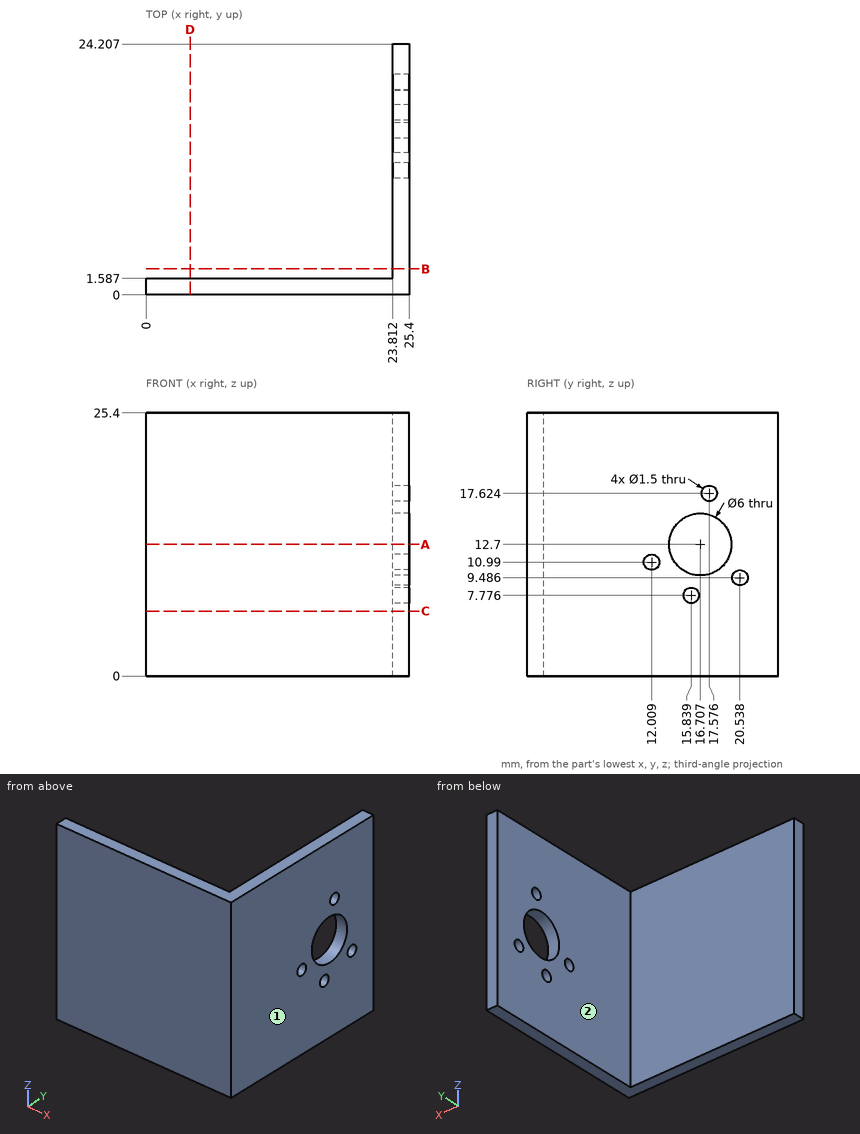
For this review, use the dimensioned drawing (mm, ordinates from the lowest corner) and the shaded views. A direction names the side the tool comes from. Coordinates: 2 decimals unless noted, no trailing zeros. Loops run counter-clockwise (first coordinate to the right, second up) from the corner with the lowest first, then second, coordinate; pieces in that order, holes last.
1. Add section A-A, the plane z = 12.7. Give the boundary of the cut face in (x, y).
2. Add section B-B, the plane y = 2.5. Give the boundary of the cut face in (x, z).
3. Add section D-D, the plane x = 4.25. Give the boundary of the cut face in (y, z).
4. Insertion check: P1, Ø11.5, axis at y = 18, z = 17, coming from the -X side; P2, Ø12, axis at x = 2.5, z = 21.5, coming from the +Y side. Each pin has a flat end and moves straight along its axis. Give the tip position at first contact, or say it passes through.
5. Add section C-C, the plane z = 6.25. Give the boundary of the cut face in (x, y).
6. For line 1 (Y direction, x = 24.6, z = 12.7); line 2 (Y direction, x = 15.5, z = 15); line 3 (X direction, y = 6.5, z = 12.75), list the stretches that pass through material, from the lowest coordinate up.
7. For the marked faces 1 and 2, list the 3-axis set-ups (+Z, -Z, +X, -X, +Y, -Y) from which the entire face can be reached by the end or side of a thin tool; tool diameter is ignored.
Result:
1. outline: (0, 0) - (25.4, 0) - (25.4, 13.71) - (23.81, 13.71) - (23.81, 1.59) - (0, 1.59) - close; (23.81, 19.71) - (25.4, 19.71) - (25.4, 24.21) - (23.81, 24.21) - close
2. outline: (23.81, 0) - (25.4, 0) - (25.4, 25.4) - (23.81, 25.4) - close
3. outline: (0, 0) - (1.59, 0) - (1.59, 25.4) - (0, 25.4) - close
4. P1: stops at x = 23.81
4. P2: stops at y = 1.59
5. outline: (0, 0) - (25.4, 0) - (25.4, 24.21) - (23.81, 24.21) - (23.81, 1.59) - (0, 1.59) - close
6. line 1: y = 0 to 13.71, 19.71 to 24.21
6. line 2: y = 0 to 1.59
6. line 3: x = 23.81 to 25.4
7. face 1: +Z, -Z, +X, +Y, -Y
7. face 2: +Z, -Z, -X, +Y
